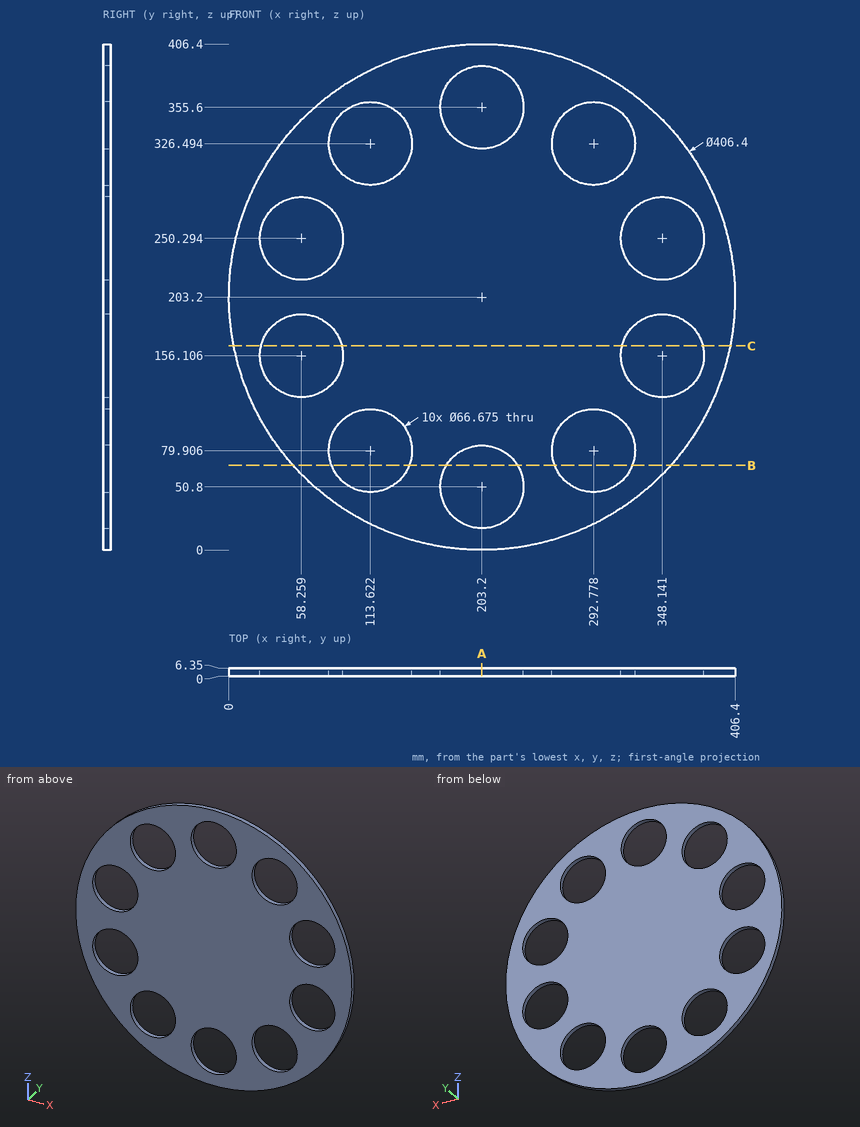
The figure shows three views and two pictorial views of one solid part (mm, origin at its lowest corner). Answer the questions. Round coordinates to 2 decimals unless told otherwise and drop trailing zeros. Loops run counter-clockwise (first coordinate to the right, second up) from the corner with the lowest first, then second, coordinate; pieces in that order, holes last. Notation, with made-up numbers: M 54.5,60.25 L 112.5,60.25 A12 ccw 112.5,82.25 Z; hole C -34,0 d10. An arc over 180 degrees is marked long. Write each question's results on one line, items separated by ' | '. Start each with the question number.
1) Straight lines are drawn through the part: probe 1 along X at (y, z) = (1, 335) (1 decimal); probe 2 along X at (y, z) = (3.5, 346.5) (1 decimal); probe 3 along Z at (x, y) = (72, 1.75) (1 decimal). For each, find the intervals that lie inside material, in ascending order.
2) Find section C-C on z = 164. Write down the section's boundary in (x, y), plus the area to 3 significant figures.
3) Find section A-A on x = 203.2. Write down the section's boundary in (y, z), plus the area to 3 significant figures.
4) Find section B-B on z = 68. Count the separate pieces of the cut face and the enclosed holes in it, plus the area to 3 significant figures.
5) Each of these flat-tipped pins is pushed along its axis until it touches: pin 1 (1 mm diameter, centred on y = 3.5, z = 284.5, fed in from -X) (1 decimal); pin 2 (2 mm diameter, centred on y = 5.5, z = 70.5, fed in from -X); pin 3 (12 mm diameter, centred on x = 111.5, z = 135, fed in from -Y). Where does it stop, or does it pass through?
Final values:
1) probe 1: 48.5 to 81.4, 145.9 to 177, 229.4 to 260.5, 325 to 357.9 | probe 2: 59.1 to 87, 140.3 to 171.1, 235.3 to 266.1, 319.4 to 347.3 | probe 3: 48 to 125.7, 186.5 to 219.9, 280.7 to 358.4
2) outline: M 3.82,0 L 25.87,0 L 25.87,6.35 L 3.82,6.35 Z; M 90.65,0 L 315.75,0 L 315.75,6.35 L 90.65,6.35 Z; M 380.53,0 L 402.58,0 L 402.58,6.35 L 380.53,6.35 Z | area: 1,710 mm²
3) outline: M 0,0 L 6.35,0 L 6.35,17.46 L 0,17.46 Z; M 0,84.14 L 6.35,84.14 L 6.35,322.26 L 0,322.26 Z; M 0,388.94 L 6.35,388.94 L 6.35,406.4 L 0,406.4 Z | area: 1,730 mm²
4) separate pieces: 4 | enclosed holes: 0 | area: 773 mm²
5) pin 1: x = 16.8 | pin 2: x = 48.46 | pin 3: y = 0
